Geometry: final body of the model. Coordinates: model frame, mm. Face numbers are marked on the shaded views. Give positions to 0.01 mm unless a question says otherwise; leave off trailing zeros. Write each loop counter-clockwise with the first axis right and the second up, starting at its lowest first coordinate (ties: lowest second). Pieces come first, ordered by that corner, then holes.
```python
from build123d import *

# Parameters (mm, degrees)
BOSS_EXTRUDE1_DEPTH = 23.8125
SKETCH2_R           = 1.905
CUT_EXTRUDE1_DEPTH  = 30.826417087
SKETCH3_R           = 1.905
CUT_EXTRUDE2_DEPTH  = 30.826417087
FILLET1_R           = 1.5875


with BuildPart() as part:
    # Sketch1 → Boss-Extrude1 (new, symmetric)
    with BuildSketch(Plane(origin=(0, 0, 0), x_dir=(1, 0, 0), z_dir=(0, 1, 0))):
        Polygon((0, 0), (-12.7, 0), (-12.7, -12.7), align=None)
    extrude(amount=BOSS_EXTRUDE1_DEPTH, both=True)

    # Sketch2 → Cut-Extrude1 (cut, through all)
    with BuildSketch(Plane.ZY.offset(12.7)):
        with Locations((6.35, 19.05)):
            Circle(SKETCH2_R)
        with Locations((6.35, -19.05)):
            Circle(SKETCH2_R)
    extrude(amount=-CUT_EXTRUDE1_DEPTH, mode=Mode.SUBTRACT)

    # Sketch3 → Cut-Extrude2 (cut, through all)
    with BuildSketch(Plane(origin=(0, 0, 0), x_dir=(-1, 0, 0), z_dir=(0, 0, -1))):
        with Locations((6.35, -12.7)):
            Circle(SKETCH3_R)
        with Locations((6.35, 12.7)):
            Circle(SKETCH3_R)
    extrude(amount=-CUT_EXTRUDE2_DEPTH, mode=Mode.SUBTRACT)

    # Fillet1
    fillet1_edges = [part.edges().sort_by_distance(p)[0] for p in [
        (-12.7, 23.8125, 6.35),
        (-12.7, -23.8125, 6.35),
        (-6.35, -23.8125, 0),
        (-6.35, -23.8125, 6.35),
        (-6.35, 23.8125, 6.35),
        (-12.7, 0, 12.7),
        (-12.7, 0, 0),
        (0, 0, 0),
        (-6.35, 23.8125, 0),
    ]]
    fillet(fillet1_edges, radius=FILLET1_R)


solid = part.part
```
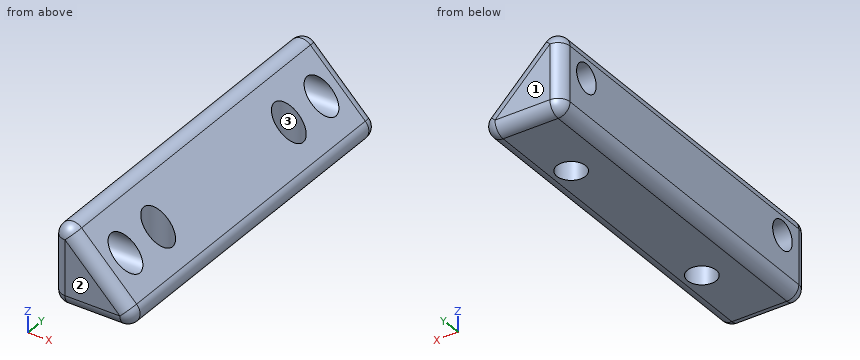
Item 1: Pin query (flat end, axial travel): pin 1 Ø1.5 at (x, y) = (-8.5, -16) entering from -Z; pin 2 Ø2 at (y, z) = (12, 8.5) entering from +X; pin 3 Ø5 at (y, z) = (-16, 9) entering from +X; pin 4 Ø2 at (y, z) = (-14, 7.5) entering from +X. Return the tip coordinate at first contact, or that it passes through.
Found:
pin 1: stops at z = 0
pin 2: stops at x = -7.72
pin 3: stops at x = -6.5
pin 4: stops at x = -6.68
Item 2: Section A-A, the plane y = 12.7. Return the cut outline in (x, z) (1 decimal).
Found:
outline: (-12.7, 1.6) arc R1.6 ccw to (-11.1, 0) - (-8.3, 0) - (-8.3, 8.3) - (-10, 10) arc R1.6 ccw to (-12.7, 8.9) - close; (-4.4, 0) - (-3.8, 0) arc R1.6 ccw to (-2.7, 2.7) - (-4.4, 4.4) - close
Item 3: Section B-B, the plane z = 7.75. State how many separate pieces and enclosed holes the cut face has, plus the area to 3 significant figures.
Found:
separate pieces: 3
enclosed holes: 0
area: 206 mm2
Item 4: Pull-direction query (Y, two-part tool) for the marked faces 1, 2 and 3; classes: +Y half, -Y half, draft (parallel to the pull), parting line (faces both ways), or undercut.
Found:
face 1: +Y half
face 2: -Y half
face 3: undercut
Item 5: Line query: L1, parallel to Y at x = -6.5, z = 2.75; L2, parallel to Y at x = -6.35, z = 5 (3 decimals); L3, parallel to Y at x = -8.75, z = 5.75. Output: solid intervals per line, ascending.
Found:
L1: y = -23.81 to -14.6, -10.8 to 10.8, 14.6 to 23.81
L2: y = -23.681 to -20.394, -17.706 to -14.605, -10.795 to 10.795, 14.605 to 17.706, 20.394 to 23.681
L3: y = -23.81 to -20.86, -17.24 to 17.24, 20.86 to 23.81
Item 6: Section D-D, the plane y = 18. Return the cut outline in (x, z) (1 decimal).
Found:
outline: (-12.7, 1.6) arc R1.6 ccw to (-11.1, 0) - (-3.8, 0) arc R1.6 ccw to (-2.7, 2.7) - (-4.8, 4.8) - (-12.7, 4.8) - close; (-12.7, 7.9) - (-7.9, 7.9) - (-10, 10) arc R1.6 ccw to (-12.7, 8.9) - close
